Verification items for the finished model (mm, model axes). Face numbers are marked on the shaded views. A direction names the side the tool comes from. Give positions to 0.01 mm unless a question says otherwise; leave off trailing zeros. Write each loop counter-clockwise with the first axis right and the second up, starting at its lowest first coordinate (ties: lowest second). Pieces come first, ordered by that corner, then holes. Notation, with made-up numbers: (-13, 81.5) - (46, 81.5) arc R9 ccw to (46, 95.5) - close; hole circle Ø2 at (63.25, -15.5). An arc over 180 degrees is marked (long way). Answer as a JSON object with one key per item and string values. Group by question number.
Item 1: Go/stop test with flat-tipped pins: pin 1 (1 mm diameter, centred on y = -1, z = 1, fed in from -X); pin 2 (0.8 mm diameter, centred on x = 0.5, z = 0.5, fed in from +Y); pin 3 (1.5 mm diameter, centred on y = 2, z = 0.5, fed in from +X). Record where each tip stops, or that it passes through.
Item 2: Sectioned sample at C-C, the plane y = -6.5. Record the boundary of the cut face in (x, z), and give its area (3 significant figures).
Item 3: Scan lines: line 1 along Z through (x, y) = (-3.25, 3.25); line 2 along Y through (x, z) = (4.25, -1.65); line 3 along X through (y, z) = (6.5, -1.3). Record each from-to range of solid material in increasing order. Write a range as [from, to].
Item 4: Sectioned sample at B-B, the plane x = 1.25. Record the boundary of the cut face in (y, z).
Item 5: Draft check along Y on the marked faces 4, 5, 6 and 7. Enter one of: +Y half, -Y half, draft (parallel to the pull), parting line (faces both ways), or undercut.
Item 6: Sectioned sample at D-D, the plane z = 1. Record the boundary of the cut face in (x, y) (3 decimals), and give its area (3 significant figures).
Item 7: Tool access check on the marked faces 1, 2 and 3. Record the directions out of +Z, -Z, +X, -X, +Y, -Y that give a thin tool (end or side, any length) a straight path to the whole face; none if there is none.
Item 8: Sectioned sample at A-A, the plane z = -1.2. Record the boundary of the cut face in (x, y), and give its area (3 significant figures).
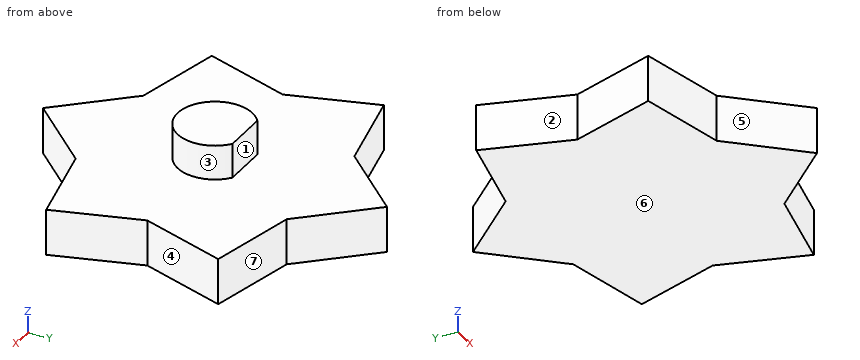
```python
from build123d import *

# Parameters (mm, degrees)
BOSS_EXTRUDE1_DEPTH      = 2
BOSS_EXTRUDE2_DEPTH      = 1.5
BOSS_EXTRUDE2_DEPTH_BACK = 2


with BuildPart() as part:
    # Sketch1 → Boss-Extrude1 (new body)
    with BuildSketch(Plane.XY):
        Polygon((0, -7.474945526), (2.647536041, -4.585666938), (6.473492718, -3.737472763), (5.295072082, 0), (6.473492718, 3.737472763), (2.647536041, 4.585666938), (0, 7.474945526), (-2.647536041, 4.585666938), (-6.473492718, 3.737472763), (-5.295072082, 0), (-6.473492718, -3.737472763), (-2.647536041, -4.585666938), align=None)
    extrude(amount=-BOSS_EXTRUDE1_DEPTH)

    # Sketch1<4> → Boss-Extrude2 (add, two sides: drawn at the far end of the back side and taken through both)
    with BuildSketch(Plane.XY.offset(-BOSS_EXTRUDE2_DEPTH_BACK)):
        with BuildLine():
            Line((0.975, 1.3), (-0.975, 1.3))
            ThreePointArc((-0.975, 1.3), (0, -1.625), (0.975, 1.3))
        make_face()
    extrude(amount=BOSS_EXTRUDE2_DEPTH + BOSS_EXTRUDE2_DEPTH_BACK)


solid = part.part
```
Geometry check:
{
 "1": {"pin 1": "x = -1.55", "pin 2": "y = 1.3", "pin 3": "x = 6.1"},
 "2": {"outline": "(-0.89, -2) - (0.89, -2) - (0.89, 0) - (-0.89, 0) - close", "area": "3.57 mm^2"},
 "3": {"line 1": "[-2, 0]", "line 2": "[-4.23, 4.23]", "line 3": "[-0.89, 0.89]"},
 "4": {"outline": "(-6.11, -2) - (6.11, -2) - (6.11, 0) - (1.04, 0) - (1.04, 1.5) - (-1.04, 1.5) - (-1.04, 0) - (-6.11, 0) - close"},
 "5": {"face 4": "undercut", "face 5": "-Y half", "face 6": "draft", "face 7": "+Y half"},
 "6": {"outline": "(-0.975, 1.3) arc R1.625 ccw (long way) to (0.975, 1.3) - close", "area": "7.86 mm^2"},
 "7": {"face 1": "+Z, +X, -X, +Y", "face 2": "+Z, -Z, -X", "face 3": "+Z"},
 "8": {"outline": "(-6.47, -3.74) - (-2.65, -4.59) - (0, -7.47) - (2.65, -4.59) - (6.47, -3.74) - (5.3, 0) - (6.47, 3.74) - (2.65, 4.59) - (0, 7.47) - (-2.65, 4.59) - (-6.47, 3.74) - (-5.3, 0) - close", "area": "119 mm^2"}
}
